Could you check a few things on this drawing? It's one solid part, dimensions in mm from its lowest x, y, z. Round coordinates to 2 decimals unless told otherwise and drop trailing zeros. Write each loop counter-clockwise with the first axis right and the second up, starting at its lowest first coordinate (ties: lowest second). Pieces come first, ordered by that corner, then holes. Notation, with made-up numbers: M 57.25,68 L 76.25,68 A4 ccw 76.25,73 Z; hole C 8.25,89 d9. An arc over 180 degrees is marked long. One line per item, written item: value. Start each with the question number.
(1) I want a section at D-D on z = 99.5. Please give me the cut outline in (x, y), and give its area (3 significant figures).
(2) I'm going to push flat-ended pins straight in: pin 1 Ø7.5 at (y, z) = (13.5, 57.5) entering from +X; pin 2 Ø9.5 at (x, z) = (288.5, 57.5) entering from +Y (3 decimals); pin 3 Ø5.5 at (y, z) = (8.5, 91) entering from -X. Where does each tip first touch, or does it pass through?
(3) I want a section at B-B on y = 14.5. Please give me the cut outline in (x, z), and give its area (3 significant figures).
(4) If I drill on L1, parallel to Z at x = 202, y = 11; L2, parallel to X at y = 12.75, z = 75.5; L3, parallel to X at y = 16.75, z = 56, over which ranges is the centre line in solid material (lowest first)?
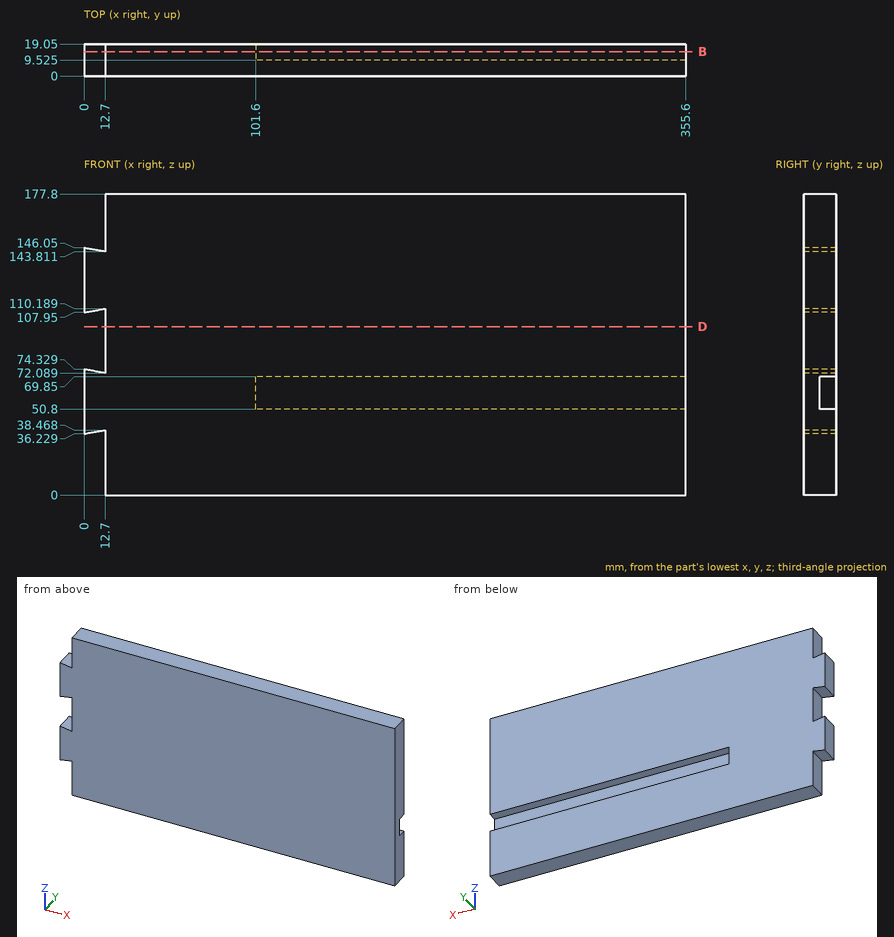
Found:
1. outline: M 12.7,0 L 355.6,0 L 355.6,19.05 L 12.7,19.05 Z
1. area: 6,530 mm²
2. pin 1: stops at x = 101.6
2. pin 2: stops at y = 9.525
2. pin 3: stops at x = 12.7
3. outline: M 0,36.23 L 12.7,38.47 L 12.7,0 L 355.6,0 L 355.6,50.8 L 101.6,50.8 L 101.6,69.85 L 355.6,69.85 L 355.6,177.8 L 12.7,177.8 L 12.7,143.81 L 0,146.05 L 0,107.95 L 12.7,110.19 L 12.7,72.09 L 0,74.33 Z
3. area: 57,000 mm²
4. L1: z = 0 to 50.8, 69.85 to 177.8
4. L2: x = 12.7 to 355.6
4. L3: x = 0 to 101.6
